Geometry: final body of the model. Coordinates: model frame, mm. Give positions to 0.01 mm unless a question says otherwise; leave off trailing zeros. Loops run counter-clockwise (first coordinate to the right, second up) from the corner with the lowest first, then second, coordinate; pieces in that order, holes last. Notation, with made-up numbers: (24.25, 65.25) -> (33.25, 65.25) arc R28 cw to (33.25, 88.25) -> close; hole circle Ø1 at (-11, 51.25). An arc over 180 degrees is marked (long way). Answer in a Markdown table with one row per item. Add a question column.
1) First-contact query: P1, Ø0.6, axis at x = -1, z = 1, coming from the +Y side. Flat tip, straight axial feed; report the tip coordinate or a pass-through.
2) Section query B-B (z = 0.3). Give the number of separate pieces and of enclosed holes in the cut face, plus the area to 3 significant figures.
3) Section query D-D (y = 27.75). Return the cut outline in (x, z), plus the area to 3 significant figures.
4) Section query C-C (x = 12). Return the cut outline in (y, z), plus the area to 3 significant figures.
5) Section query A-A (y = -4). Return the cut outline in (x, z).
6) Line query: line 1 (Y direction, x = 0, z = 0.75); line 2 (X direction, y = -4.5, z = 0.7); line 3 (X direction, y = 11, z = 1.2). Output: solid intervals per line, ascending. Write a range as from..to.
```python
from build123d import *

# Parameters (mm, degrees)
F0_R     = 1.5
F0_R_2   = 3.25
F1_DEPTH = 2
F2_R     = 3
F3_W     = 12
F3_H     = 17
F4_DEPTH = 25
F5_R     = 1


with BuildPart() as f1:
    # F0 (on Top) → F1 (new body)
    with BuildSketch(Plane.XY):
        with BuildLine():
            Line((-15.5, 14.0758867192), (-15.5, -14.0758867192))
            ThreePointArc((-15.5, -14.0758867192), (-9.9776979071, -20.6460779619), (-6.0661514917, -28.2856485004))
            ThreePointArc((-6.0661514917, -28.2856485004), (0, -32.4824673534), (6.0661514917, -28.2856485004))
            ThreePointArc((6.0661514917, -28.2856485004), (9.9776979071, -20.6460779619), (15.5, -14.0758867192))
            Line((15.5, -14.0758867192), (15.5, 14.0758867192))
            ThreePointArc((15.5, 14.0758867192), (9.4126848848, 21.5229485882), (5.3843378024, 30.2571661019))
            Line((5.3843378024, 30.2571661019), (4.948926344, 30.8923631943))
            ThreePointArc((4.948926344, 30.8923631943), (0, 33.5), (-4.948926344, 30.8923631943))
            Line((-4.948926344, 30.8923631943), (-5.3843378024, 30.2571661019))
            ThreePointArc((-5.3843378024, 30.2571661019), (-9.4126848848, 21.5229485882), (-15.5, 14.0758867192))
        make_face()
        with Locations((0, -26)):
            Circle(F0_R, mode=Mode.SUBTRACT)
        with Locations((-12, 0)):
            Circle(F0_R, mode=Mode.SUBTRACT)
        with Locations((12, 0)):
            Circle(F0_R, mode=Mode.SUBTRACT)
        with Locations((-12, 12)):
            Circle(F0_R, mode=Mode.SUBTRACT)
        with Locations((0, 27.75)):
            Circle(F0_R_2, mode=Mode.SUBTRACT)
        with Locations((12, 12)):
            Circle(F0_R, mode=Mode.SUBTRACT)
    extrude(amount=F1_DEPTH)

    # F2
    f2_edges = [f1.edges().sort_by_distance(p)[0] for p in [
        (-15.5, 14.075887, 1),
        (5.384338, 30.257166, 1),
        (-5.384338, 30.257166, 1),
        (-15.5, -14.075887, 1),
        (15.5, -14.075887, 1),
        (15.5, 14.075887, 1),
    ]]
    fillet(f2_edges, radius=F2_R)

    # F3 (on face) → F4 (cut)
    with BuildSketch(Plane.XY.offset(2)):
        with Locations((0, -8)):
            Rectangle(F3_W, F3_H)
    extrude(amount=-F4_DEPTH, mode=Mode.SUBTRACT)

    # F5
    f5_edges = [f1.edges().sort_by_distance(p)[0] for p in [
        (-6, 0.5, 1),
        (6, 0.5, 1),
        (6, -16.5, 1),
        (-6, -16.5, 1),
    ]]
    fillet(f5_edges, radius=F5_R)


solid = f1.part
```
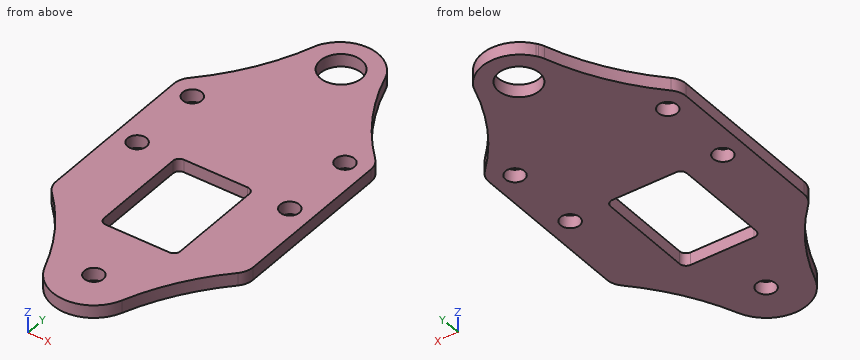
Evaluation:
| question | item | result |
|---|---|---|
| 1 | P1 | y = 33.46 |
| 2 | separate pieces | 1 |
| 2 | enclosed holes | 7 |
| 2 | area | 1,250 mm² |
| 3 | outline | (-6.27, 0) -> (-3.25, 0) -> (-3.25, 2) -> (-6.27, 2) -> close; (3.25, 0) -> (6.27, 0) -> (6.27, 2) -> (3.25, 2) -> close |
| 3 | area | 12.1 mm² |
| 4 | outline | (-17.88, 0) -> (-1.5, 0) -> (-1.5, 2) -> (-17.88, 2) -> close; (1.5, 0) -> (10.5, 0) -> (10.5, 2) -> (1.5, 2) -> close; (13.5, 0) -> (17.88, 0) -> (17.88, 2) -> (13.5, 2) -> close |
| 4 | area | 59.5 mm² |
| 5 | outline | (-15.5, 0) -> (-6, 0) -> (-6, 2) -> (-15.5, 2) -> close; (6, 0) -> (15.5, 0) -> (15.5, 2) -> (6, 2) -> close |
| 6 | line 1 | -32.48..-27.5, -24.5..-16.5, 0.5..24.5, 31..33.5 |
| 6 | line 2 | -15.5..-6, 6..15.5 |
| 6 | line 3 | -15.5..-13.12, -10.88..10.88, 13.12..15.5 |
